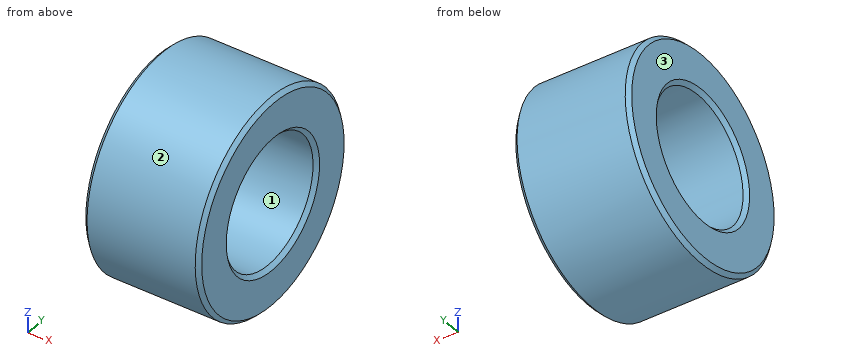
from build123d import *

# Parameters (mm, degrees)
SKETCH1_R          = 55
SKETCH1_R_2        = 30
EXTRUDE1_DEPTH     = 30
SKETCH2_R          = 32.75
MACHINE_DEPTH      = 30
CHAMFER_OUTER_SIZE = 2
CHAMFER_INNER_SIZE = 2


with BuildPart() as part:
    # Sketch1 → Extrude1 (new body, symmetric)
    with BuildSketch(Plane(origin=(0, 0, 0), x_dir=(0, 0, -1), z_dir=(1, 0, 0))):
        Circle(SKETCH1_R)
        Circle(SKETCH1_R_2, mode=Mode.SUBTRACT)
    extrude(amount=EXTRUDE1_DEPTH, both=True)

    # Sketch2 → Machine (cut, symmetric)
    with BuildSketch(Plane(origin=(0, 0, 0), x_dir=(0, 0, -1), z_dir=(1, 0, 0))):
        Circle(SKETCH2_R)
    extrude(amount=MACHINE_DEPTH, both=True, mode=Mode.SUBTRACT)

    # Chamfer-Outer
    chamfer_outer_edges = [part.edges().sort_by_distance(p)[0] for p in [
        (30, 0, 55),
        (-30, 0, 55),
    ]]
    chamfer(chamfer_outer_edges, length=CHAMFER_OUTER_SIZE)

    # Chamfer-Inner
    chamfer_inner_edges = [part.edges().sort_by_distance(p)[0] for p in [
        (30, 0, 32.75),
        (-30, 0, 32.75),
    ]]
    chamfer(chamfer_inner_edges, length=CHAMFER_INNER_SIZE)


solid = part.part
Here's how the part is built. I have some questions about the finished solid (model axes, mm). Face numbers are marked on the shaded views. Round coordinates to 2 decimals unless told otherwise and drop trailing zeros. Loops run counter-clockwise (first coordinate to the right, second up) from the corner with the lowest first, then second, coordinate; pieces in that order, holes last. Notation, with made-up numbers: M 44,-35.75 L 50,-35.75 A13 ccw 50,-24.75 Z; hole C 32,0.5 d10. An arc over 180 degrees is marked long. Write each question's results on one line, items separated by ' | '. Start each with the question number.
(1) Will these pins go through, and if not, where does the flat tip stop? P1, Ø3, axis at x = -4, z = -15, coming from the +Y side; P2, Ø8, axis at x = 8.5, z = 36, coming from the -Y side; P3, Ø8, axis at x = 0.5, z = -6.5, coming from the +Y side.
(2) I want a section at C-C (x = 11). Please give me the cut outline in (y, z), then the cut area to 3 significant figures.
(3) If I drill on probe 1 along Y at (x, z) = (5.5, 0); probe 2 along Z at (x, y) = (4.5, 7.5); probe 3 along Y at (x, z) = (-3, 11.5), over which ranges is the centre line in solid material (lowest first)? Write a range as from..to.
(4) Thinking about a two-plate mould opening in Z: for the marked faces 1, 2 and 3, which applies, pulls with the +Z half, pulls with the -Z half, needs draft (parallel to the pull), parting line crosses it, or undercut?
(5) I want a section at A-A (y = 0). Please give me the cut outline in (x, z).
Solved:
1) P1: stops at y = 53.32 | P2: stops at y = -44.73 | P3: stops at y = 54.94
2) outline: C 0,0 d110; hole C 0,0 d65.5 | area: 6,130 mm²
3) probe 1: y = -55..-32.75, 32.75..55 | probe 2: z = -54.49..-31.88, 31.88..54.49 | probe 3: y = -53.78..-30.66, 30.66..53.78
4) face 1: undercut | face 2: parting line crosses it | face 3: needs draft
5) outline: M -30,-53 L -28,-55 L 28,-55 L 30,-53 L 30,-34.75 L 28,-32.75 L -28,-32.75 L -30,-34.75 Z; M -30,34.75 L -28,32.75 L 28,32.75 L 30,34.75 L 30,53 L 28,55 L -28,55 L -30,53 Z
